from build123d import *

# Parameters (mm, degrees)
SKETCH1_W           = 114
SKETCH1_H           = 74
BOSS_EXTRUDE1_DEPTH = 40
SHELL1_T            = -2
SKETCH2_W           = 8
SKETCH2_H           = 3.224245312
BOSS_EXTRUDE2_DEPTH = 12
CUT_EXTRUDE1_REACH  = 89.92
SKETCH3_W           = 93.912635184
SKETCH3_H           = 51.017060478
SKETCH4_W           = 51.053224202
SKETCH4_H           = 19.102136622
CUT_EXTRUDE2_DEPTH  = 138.277092044
SKETCH5_W           = 92.288442818
SKETCH5_H           = 29.598231076
CUT_EXTRUDE3_DEPTH  = 109.797977922
SKETCH6_W           = 4.328253691
SKETCH6_H           = 19.102136622
CUT_EXTRUDE4_DEPTH  = 12
FILLET1_R           = 3
SKETCH7_R           = 1.3
CUT_EXTRUDE5_DEPTH  = 12


with BuildPart() as part:
    # Sketch1 → Boss-Extrude1 (new body)
    with BuildSketch(Plane(origin=(0, 0, 0), x_dir=(1, 0, 0), z_dir=(0, 1, 0))):
        Rectangle(SKETCH1_W, SKETCH1_H)
    extrude(amount=BOSS_EXTRUDE1_DEPTH)

    # Shell1
    shell1_openings = [part.faces().sort_by_distance(p)[0] for p in [
        (0, 0, 0),
    ]]
    offset(amount=SHELL1_T, openings=shell1_openings, kind=Kind.INTERSECTION)

    # Sketch2 → Boss-Extrude2 (add)
    with BuildSketch(Plane.ZY.offset(57)):
        with Locations((-33, 1.612122656)):
            Rectangle(SKETCH2_W, SKETCH2_H)
        with Locations((33, 1.612122656)):
            Rectangle(SKETCH2_W, SKETCH2_H)
    boss_extrude2 = extrude(amount=BOSS_EXTRUDE2_DEPTH)

    # Mirror1: Boss-Extrude2 across plane
    add(boss_extrude2.mirror(Plane.ZY))

    # Sketch3 → Cut-Extrude1 (cut, up to next)
    with BuildSketch(Plane(origin=(0, 40, 0), x_dir=(1, 0, 0), z_dir=(0, 1, 0)), mode=Mode.PRIVATE) as cut_extrude1_sk1:
        with Locations((0.781529231, 0.507308448)):
            Rectangle(SKETCH3_W, SKETCH3_H)
    cut_extrude1_tool1 = extrude(cut_extrude1_sk1.sketch, amount=-CUT_EXTRUDE1_REACH, mode=Mode.PRIVATE) & part.part
    add(cut_extrude1_tool1.solids().sort_by_distance((0.781529, 40, -0.507308))[0], mode=Mode.SUBTRACT)

    # Sketch4 → Cut-Extrude2 (cut, through all)
    with BuildSketch(Plane.ZY.offset(57)):
        with Locations((0.2378186, 20.916211941)):
            Rectangle(SKETCH4_W, SKETCH4_H)
    extrude(amount=-CUT_EXTRUDE2_DEPTH, mode=Mode.SUBTRACT)

    # Sketch5 → Cut-Extrude3 (cut, through all)
    with BuildSketch(Plane.XY.offset(37)):
        with Locations((1, 20)):
            Rectangle(SKETCH5_W, SKETCH5_H)
    extrude(amount=-CUT_EXTRUDE3_DEPTH, mode=Mode.SUBTRACT)

    # Sketch6 → Cut-Extrude4 (cut)
    with BuildSketch(Plane.ZY.offset(57)):
        with Locations((27.928557547, 20.916211941)):
            Rectangle(SKETCH6_W, SKETCH6_H)
    extrude(amount=-CUT_EXTRUDE4_DEPTH, mode=Mode.SUBTRACT)

    # Fillet1
    fillet1_edges = [part.edges().sort_by_distance(p)[0] for p in [
        (47.144221409, 34.799115538, -36),
        (47.144221409, 5.200884462, -36),
        (-45.144221409, 5.200884462, -36),
        (-45.144221409, 34.799115538, -36),
        (47.144221409, 34.799115538, 36),
        (47.144221409, 5.200884462, 36),
        (-45.144221409, 5.200884462, 36),
        (-45.144221409, 34.799115538, 36),
        (-56, 30.467280252, 30.092684392),
        (-56, 11.36514363, 30.092684392),
        (55, 19, 35),
        (55, 19, -35),
        (-55, 19, -35),
        (-55, 19, 35),
        (55, 38, 0),
        (0, 38, -35),
        (-55, 38, 0),
        (0, 38, 35),
        (-57, 3.224245312, -33),
        (-57, 3.224245312, 33),
        (57, 3.224245312, -33),
        (57, 3.224245312, 33),
        (-46.174788361, 39, 25.001221791),
        (-46.174788361, 39, -26.015838687),
        (47.737846823, 39, -26.015838687),
        (47.737846823, 39, 25.001221791),
        (56, 30.467280252, 25.764430701),
        (56, 11.36514363, 25.764430701),
        (56, 11.36514363, -25.288793501),
        (56, 30.467280252, -25.288793501),
        (-56, 11.36514363, -25.288793501),
        (-56, 30.467280252, -25.288793501),
    ]]
    fillet(fillet1_edges, radius=FILLET1_R)

    # Sketch7 → Cut-Extrude5 (cut)
    with BuildSketch(Plane.XZ):
        with Locations(Location((-63.1, -32.825, 0), (0, 0, 270))):
            Circle(SKETCH7_R)
        with Locations(Location((-63.1, 32.825, 0), (0, 0, 270))):
            Circle(SKETCH7_R)
        with Locations(Location((63.1, 32.825, 0), (0, 0, 270))):
            Circle(SKETCH7_R)
        with Locations(Location((63.1, -32.825, 0), (0, 0, 270))):
            Circle(SKETCH7_R)
    extrude(amount=-CUT_EXTRUDE5_DEPTH, mode=Mode.SUBTRACT)


solid = part.part
Here's how the part is built. I have some questions about the finished solid (model axes, mm). A direction names the side the tool comes from. Give positions to 0.01 mm unless a question says otherwise; leave off trailing zeros. Order: outer loops, then holes, each group sorted by start corner. A loop starts at its lowest first (then second) coordinate and runs counter-clockwise, first axis right, second up. Notation, with made-up numbers: M -27,-19.5 L -4,-19.5 A18 ccw -4,-14.5 Z; hole C 4.25,13 d8. An arc over 180 degrees is marked long. Answer as a JSON object with one key per item and string values. Group by question number.
1) On a 3-axis mill with a long thin cutter (end or side, diameter ignored), from which of +Z, -Z, +X, -X, +Y, -Y can I reach the whole of each face in a straight line? I mean faces 1 (the flat face through (63, 2, 29)), 2 (the cylindrical face through (46.242, 6.056, 35.986)), 3 (the flat face through (-64, 3.224, -34)). Say none if no direction works.
2) Suppose I cut it at A-A, the plane y = 17.5. Write out the boundary of the cut face in (x, z), plus the area to 3 significant figures.
3) Suppose I cut it at B-B, the plane x = 38.5. Write out the boundary of the cut face in (y, z).
4) Suppose I cut it at C-C, the plane z = 6. Write out the boundary of the cut face in (x, y).
5) Suppose I cut it at D-D, the plane z = -27.5. Write out the boundary of the cut face in (x, y).
6) I'm going to push flat-ended pins straight in: pin 1 Ø12 at (y, z) = (5.5, -7.5) entering from +X; pin 2 Ø0.6 at (y, z) = (22.5, 36) entering from -X; pin 3 Ø3 at (x, z) = (63.1, 32.825) entering from +Y. Where does each tip first touch, or does it pass through?
7) Please list where these lines run through material, in increasing order: L1, parallel to X at y = 5, z = 20; L2, parallel to X at y = 2, z = -30; L3, parallel to X at y = 19, z = 27. Write a range as [from, to].
8) We'd pull the mould along X, two halves only. Please class faces 4 (the cylindrical face through (56, 29.6, -24.4)), 5 (the flat face through (57, 11, 1)), 6 (the cylindrical face through (-54.1, 17.26, -34.14)), 7 (the cylindrical face through (54.14, 37.1, -0.45)): pulls with the +X half, pulls with the -X half, needs draft (parallel to the pull), parting line crosses it, or undercut.
Results found:
{
 "1": {"face 1": "+X, +Y, -Y", "face 2": "+Z, -Z", "face 3": "+Z, -Z, -X, +Y"},
 "2": {"outline": "M -57,-37 L -45.14,-37 L -45.14,-35 L -52,-35 A3 cw -55,-32 L -55,-25.29 L -57,-25.29 Z; M -57,30.09 L -55,30.09 L -55,32 A3 cw -52,35 L -45.14,35 L -45.14,37 L -57,37 Z; M 47.14,-37 L 57,-37 L 57,-25.29 L 55,-25.29 L 55,-32 A3 cw 52,-35 L 47.14,-35 Z; M 47.14,35 L 52,35 A3 cw 55,32 L 55,25.76 L 57,25.76 L 57,37 L 47.14,37 Z", "area": "162 mm²"},
 "3": {"outline": "M 0,-37 L 5.2,-37 L 5.2,-35 L 0,-35 Z; M 0,35 L 5.2,35 L 5.2,37 L 0,37 Z; M 34.8,-37 L 40,-37 L 40,-26.02 L 38,-26.02 L 38,-32 A3 cw 35,-35 L 34.8,-35 Z; M 34.8,35 L 35,35 A3 cw 38,32 L 38,25 L 40,25 L 40,37 L 34.8,37 Z"},
 "4": {"outline": "M -57,0 L -55,0 L -55,11.37 L -57,11.37 Z; M -57,30.47 L -55,30.47 L -55,35 A3 cw -52,38 L -46.17,38 L -46.17,40 L -57,40 Z; M 47.74,38 L 52,38 A3 cw 55,35 L 55,30.47 L 57,30.47 L 57,40 L 47.74,40 Z; M 55,0 L 57,0 L 57,11.37 L 55,11.37 Z"},
 "5": {"outline": "M -57,0 L -55,0 L -55,35 A3 cw -52,38 L 52,38 A3 cw 55,35 L 55,0 L 57,0 L 57,40 L -57,40 Z"},
 "6": {"pin 1": "x = 57", "pin 2": "x = -57", "pin 3": "y = 3.22"},
 "7": {"L1": "[-57, -55], [55, 57]", "L2": "[-69, -55], [55, 69]", "L3": "[55, 57]"},
 "8": {"face 4": "needs draft", "face 5": "pulls with the +X half", "face 6": "undercut", "face 7": "undercut"}
}
